from build123d import *

# Parameters (mm, degrees)
F0_W     = 89.9249566834
F0_H     = 150
F1_ANGLE = 45
F2_T     = -20
F3_R     = 7.5
F4_DEPTH = 15
F4_TAPER = 8
F5_R     = 7.5
F6_DEPTH = 15
F6_TAPER = 8
F7_R     = 9.99999


# Not quite as in the source:
# - a fillet or chamfer is up to 0.001 mm smaller than in the source, because OpenCascade refuses the exact size
# - a feature names something its author has since deleted; it is built from what else it names


with BuildPart() as f1:
    # F0 (on Front) → F1 (revolve)
    with BuildSketch(Plane.XZ):
        with Locations((82.3541893682, 224.1176688539)):
            Rectangle(F0_W, F0_H)
    revolve(axis=Axis((127.3166677099, 0, 224.1176688539), (0, 0, -1)), revolution_arc=F1_ANGLE)

    # F2
    f2_openings = [f1.faces().sort_by_distance(p)[0] for p in [
        (82.354189, 0, 224.117669),
        (95.523394, 31.793273, 224.117669),
        (73.342731, 22.356737, 149.117669),
        (73.342731, 22.356737, 299.117669),
    ]]
    offset(amount=F2_T, openings=f2_openings)

    # F3 (on face) → F4 (join)
    with BuildSketch(Plane.XZ):
        with Locations((47.3917110264, 219.1176688539)):
            Circle(F3_R)
    extrude(amount=F4_DEPTH, taper=F4_TAPER)

    # F5 (on face) → F6 (cut)
    with BuildSketch(Plane(origin=(63.6583338549, 63.6583338549, 0), x_dir=(-0.7071067812, 0.7071067812, 0), z_dir=(0.7071067812, 0.7071067812, 0))):
        with Locations((-9.8187575006, 219.1176688539)):
            Circle(F5_R)
    extrude(amount=-F6_DEPTH, taper=F6_TAPER, mode=Mode.SUBTRACT)

    # F7 (radius 10 in the source; OpenCascade refuses exactly that, so slightly less here)
    f7_edges = [f1.edges().sort_by_distance(p)[0] for p in [
        (44.236841, 34.412791, 299.117669),
        (62.714431, 26.759122, 299.117669),
    ]]
    fillet(f7_edges, radius=F7_R)


solid = f1.part
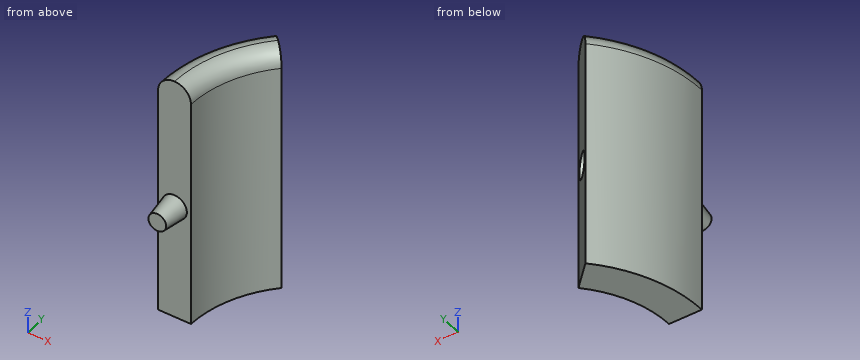
Read the model definition and answer for the solid it produces. Units are mm, in the model's axes. Coordinates: 2 decimals unless noted, no trailing zeros. Order: outer loops, then holes, each group sorted by start corner. A loop starts at its lowest first (then second) coordinate and runs counter-clockwise, first axis right, second up. Notation, with made-up numbers: (83, 44.5) -> (115, 44.5) arc R25 cw to (115, 68.5) -> close; hole circle Ø10 at (-6.5, 55). An arc over 180 degrees is marked (long way). Answer as a JSON object with one key per item and string values.
1) Consider line 1 along X through (y, z) = (23, 229.5); line 2 along Y through (x, z) = (70.5, 188); line 3 along X through (y, z) = (8, 168). Determine where each line is inside the solid, lowest interval first. Write a range as from..to.
Model answer:
{"line 1": "x = 40.38..61.28", "line 2": "y = 40.76..56.82", "line 3": "x = 37.75..57.85"}
2) Each of these flat-tipped pins is pushed along its axis until it touches: pin 1 (5 mm diameter, centred on y = 2.5, z = 210, fed in from +X); pin 2 (3 mm diameter, centred on y = 28.5, z = 205.5, fed in from -X); pin 3 (4 mm diameter, centred on y = 27, z = 239, fed in from -X). Where does it stop, or does it pass through?
Model answer:
{"pin 1": "stops at x = 57.57", "pin 2": "stops at x = 41.54", "pin 3": "stops at x = 40.94"}
3) A cutting plane is placed at A-A, the plane z = 203.5. Determine the outline of the cut face in (x, y), plus the area to 3 significant figures.
Model answer:
{"outline": "(37.39, 0) -> (57.39, 0) arc R69.92 cw to (77.87, 49.44) -> (63.73, 63.59) arc R89.92 ccw to start", "area": "1,260 mm²"}
